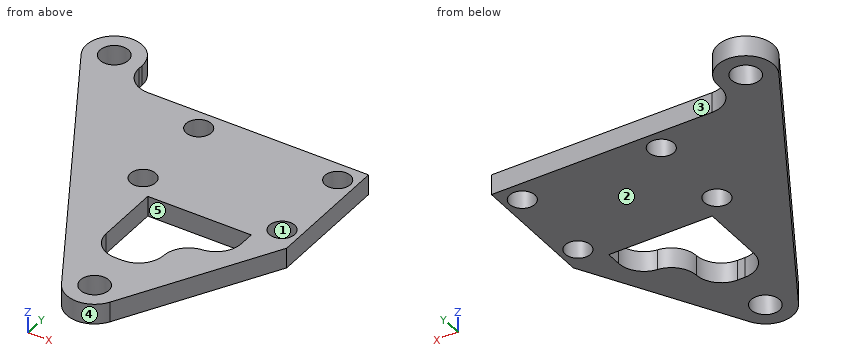
Autodesk Inventor part; units mm, degrees
ref_plane "YZ Plane" through (0, 0, 0) normal (1, 0, 0) x (0, 1, 0)
ref_plane "XZ Plane" through (0, 0, 0) normal (0, 1, 0) x (-1, 0, 0)
ref_plane "XY Plane" through (0, 0, 0) normal (0, 0, 1) x (1, 0, 0)
sketch "Sketch1" plane through (0, 0, 0) normal (0, 0, 1) x (1, 0, 0)
  circle A0 centre (0, 0) radius 3.4925
  circle A1 centre (-20.955, 36.2951) radius 3.4925
  line L0 (0, 0) -> (-43.0857, 0) construction
  circle A2 centre (-20.955, 36.2951) radius 1.778
  circle A3 centre (0, 0) radius 1.778
  line L1 (-17.4625, 36.2951) -> (-17.4625, 32.4851)
  line L2 (-17.4625, 32.4851) -> (13.335, 32.4851)
  line L3 (13.335, 32.4851) -> (13.335, 16.6101)
  line L4 (13.335, 16.6101) -> (3.0451, -1.7103)
  line L5 (-23.9796, 34.5489) -> (-3.0246, -1.7463)
  dimension "d0" = 6.985
  dimension "d1" = 6.985
  dimension "d2" = 41.91
  dimension "d3" = 60
  dimension "d5" = 3.556
  dimension "d6" = 3.556
  dimension "d7" = 3.81
  dimension "d8" = 34.29
  dimension "d29" = 15.875
extrude "Extrusion1" add sketch "Sketch1" along normal blind 2.54
sketch "Sketch3" plane through (0, 0, 2.54) normal (0, 0, 1) x (1, 0, 0)
  circle A0 centre (-20.955, 36.2951) radius 1.778 construction
  circle A1 centre (0, 0) radius 1.778 construction
  arc A2 (-3.0246, -1.7463) -> (3.0451, -1.7103) centre (0, 0) ccw construction
  line L0 (3.0451, -1.7103) -> (13.335, 16.6101) construction
  line L1 (13.335, 16.6101) -> (13.335, 32.4851) construction
  line L2 (13.335, 32.4851) -> (-17.4625, 32.4851) construction
  line L3 (-17.4625, 32.4851) -> (-17.4625, 36.2951) construction
  arc A3 (-17.4625, 36.2951) -> (-23.9796, 34.5489) centre (-20.955, 36.2951) ccw construction
  line L4 (-23.9796, 34.5489) -> (-3.0246, -1.7463) construction
  line L5 (13.335, 16.6101) -> (13.335, 32.4851)
  line L6 (13.335, 32.4851) -> (8.89, 32.4851)
  line L7 (8.89, 32.4851) -> (8.89, 16.6101)
  line L8 (8.89, 16.6101) -> (13.335, 16.6101)
  line L9 (13.335, 16.6101) -> (13.335, 32.4851)
  line L10 (-4.064, 32.4851) -> (-8.509, 32.4851)
  line L11 (-8.509, 32.4851) -> (-8.509, 16.6101)
  line L12 (-8.509, 16.6101) -> (-4.064, 16.6101)
  line L13 (-4.064, 16.6101) -> (-4.064, 32.4851)
  line L14 (8.89, 16.6101) -> (-4.064, 16.6101) construction
  dimension "d11" = 4.445
  dimension "d12" = 12.954
extrude "Extrusion2" add sketch "Sketch3" along normal blind 5.334
fillet "Fillet1" radius 3.175 1 edges at (-17.4625, 32.4851, 1.27)
sketch "Sketch4" plane through (0, 0, 2.54) normal (0, 0, 1) x (1, 0, 0)
  line L0 (-4.064, 32.4851) -> (-4.064, 16.6101)
  line L1 (-4.064, 16.6101) -> (8.89, 16.6101)
  line L2 (8.89, 16.6101) -> (8.89, 11.5301)
  line L3 (8.89, 11.5301) -> (-4.064, 11.5301)
  line L4 (-4.064, 11.5301) -> (-4.064, 16.6101)
  line L5 (-4.064, 11.5301) -> (3.175, 11.5301)
  line L6 (3.175, 11.5301) -> (3.175, 5.3796)
  line L7 (3.175, 5.3796) -> (-4.064, 5.3796)
  line L8 (-4.064, 5.3796) -> (-4.064, 11.5301)
  point P0 (0, 0)
  dimension "d16" = 5.08
  dimension "d17" = 7.239
extrude "Extrusion3" cut sketch "Sketch4" against normal through all
fillet "Fillet2" radius 3.175 4 edges at (8.89, 11.5301, 1.27) (3.175, 5.3796, 1.27) (-4.064, 5.3796, 1.27) (3.175, 11.5301, 1.27)
sketch "Sketch5" plane through (0, 0, 7.874) normal (0, 0, 1) x (1, 0, 0)
  circle A0 centre (-6.2865, 29.9451) radius 1.5875
  circle A1 centre (-6.2865, 19.1501) radius 1.5875
  circle A2 centre (11.1125, 29.9451) radius 1.5875
  circle A3 centre (11.1125, 19.1501) radius 1.5875
  line L0 (-4.064, 32.4851) -> (-8.509, 32.4851) construction
  line L1 (-8.509, 32.4851) -> (-8.509, 16.6101) construction
  line L2 (-8.509, 16.6101) -> (-4.064, 16.6101) construction
  line L3 (-4.064, 16.6101) -> (-4.064, 32.4851) construction
  line L4 (13.335, 32.4851) -> (8.89, 32.4851) construction
  line L5 (8.89, 32.4851) -> (8.89, 16.6101) construction
  line L6 (8.89, 16.6101) -> (13.335, 16.6101) construction
  line L7 (13.335, 16.6101) -> (13.335, 32.4851) construction
  point P0 (0, 0)
  point P1 (-6.2865, 32.4851)
  point P2 (11.1125, 32.4851)
  dimension "d21" = 3.175
  dimension "d22" = 3.175
  dimension "d23" = 3.175
  dimension "d24" = 3.175
  dimension "d25" = 2.54
  dimension "d26" = 2.54
extrude "Extrusion4" cut sketch "Sketch5" against normal through all
sketch "Sketch7" plane through (0, 0, 2.54) normal (0, 0, 1) x (1, 0, 0)
  line L0 (-34.1743, 47.2868) -> (24.1681, 47.2868)
  line L1 (24.1681, 47.2868) -> (24.1681, -8.7063)
  line L2 (24.1681, -8.7063) -> (-34.1743, -8.7063)
  line L3 (-34.1743, -8.7063) -> (-34.1743, 47.2868)
  point P0 (0, 0)
extrude "Extrusion6" cut sketch "Sketch7" along normal blind 25.4
properties part number "ribbonCableMount2"
Here's how the part is built. I have some questions about the finished solid (model axes, mm). Face numbers are marked on the shaded views. A direction names the side the tool comes from. Coordinates: 2 decimals unless noted, no trailing zeros. Write each loop counter-clockwise with the first axis right and the second up, starting at its lowest first coordinate (ties: lowest second). Pieces come first, ordered by that corner, then holes.
1) If I drill on line 1 (Y direction, x = -1.5, z = 1.75); line 2 (Y direction, x = -5, z = 0.55) (3 decimals); line 3 (X direction, y = 7, z = 1.45), over which ranges is the centre line in solid material (lowest first)?
Filled in:
line 1: y = -3.15 to -0.95, 0.95 to 5.44, 16.61 to 32.49
line 2: y = 1.675 to 18.22, 20.08 to 29.015, 30.875 to 32.485
line 3: x = -8.07 to -3.66, 2.77 to 7.94
2) Which directions (+Z, -Z, +X, -X, +Y, -Y) give clear straight access to the entire face, cutting with the end or side of a thin tool? Please do the marked faces 4 and 5.
Filled in:
face 4: +Z, -Z, -Y
face 5: +Z, -Z
3) I'm going to push a flat-ended pin straight in: pin 1 (1 mm diameter, centred on x = 8, z = 1.5, fed in from +Y). Where does the tip first touch, or does it pass through?
Filled in:
pin 1: stops at y = 32.49
4) If we section it at C-C (x = 2.5): List the corners of the cut face in (y, z) for me.
Filled in:
outline: (-2.44, 0) - (6.6, 0) - (6.6, 2.54) - (-2.44, 2.54) - close; (16.61, 0) - (32.49, 0) - (32.49, 2.54) - (16.61, 2.54) - close
5) If we section it at D-D (z = 0.55): Count the separate pieces of the cut face and the enclosed holes in it, plus the area to 3 significant figures.
Filled in:
separate pieces: 1
enclosed holes: 7
area: 699 mm2
6) If we section it at B-B (y = 7): List the corners of the cut face in (x, z) for me.
Filled in:
outline: (-8.07, 0) - (-3.66, 0) - (-3.66, 2.54) - (-8.07, 2.54) - close; (2.77, 0) - (7.94, 0) - (7.94, 2.54) - (2.77, 2.54) - close
7) If we section it at A-A (x = -7): List the corners of the cut face in (y, z) for me.
Filled in:
outline: (5.14, 0) - (17.73, 0) - (17.73, 2.54) - (5.14, 2.54) - close; (20.57, 0) - (28.53, 0) - (28.53, 2.54) - (20.57, 2.54) - close; (31.36, 0) - (32.49, 0) - (32.49, 2.54) - (31.36, 2.54) - close
8) Thinking about a two-plate mould opening in Y: for the marked faces 1, 2 and 3, which applies, +Y half, -Y half, draft (parallel to the pull), parting line (faces both ways), or undercut?
Filled in:
face 1: undercut
face 2: draft
face 3: +Y half
